The model under review builds one solid part; all positions refer to its coordinate system, in mm. Face numbers are marked on the shaded views. Give positions to 0.01 mm unless a question says otherwise; leave off trailing zeros. Order: outer loops, then holes, each group sorted by start corner. A loop starts at its lowest first (then second) coordinate and runs counter-clockwise, first axis right, second up. Notation, with made-up numbers: (-40, 72.25) - (14, 72.25) arc R23 cw to (14, 105.25) - close; hole circle Ø9 at (80, -26.75). An arc over 180 degrees is marked (long way). Answer as CSV lines item,"result". Start each with the question number.
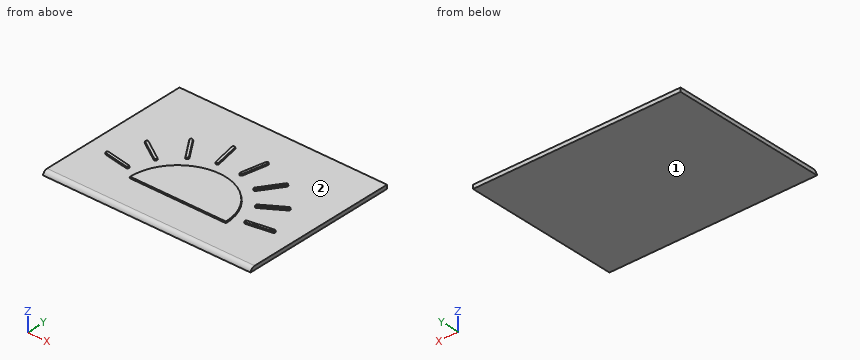
from build123d import *

# Parameters (mm, degrees)
SKETCH1_W                     = 129
SKETCH1_H                     = 97
BOSS_EXTRUDE1_DEPTH           = 2.4
FILLET1_R                     = 3
BOSS_EXTRUDE2_DEPTH           = 0.8
BOSS_EXTRUDE2_DRAFT           = 15
BOSS_EXTRUDE2_PROFILE_2_DEPTH = 0.8
BOSS_EXTRUDE2_PROFILE_2_DRAFT = 15
BOSS_EXTRUDE2_PROFILE_3_DEPTH = 0.8
BOSS_EXTRUDE2_PROFILE_3_DRAFT = 15
BOSS_EXTRUDE2_PROFILE_4_DEPTH = 0.8
BOSS_EXTRUDE2_PROFILE_4_DRAFT = 15
BOSS_EXTRUDE2_PROFILE_5_DEPTH = 0.8
BOSS_EXTRUDE2_PROFILE_5_DRAFT = 15
BOSS_EXTRUDE2_PROFILE_6_DEPTH = 0.8
BOSS_EXTRUDE2_PROFILE_6_DRAFT = 15
BOSS_EXTRUDE2_PROFILE_7_DEPTH = 0.8
BOSS_EXTRUDE2_PROFILE_7_DRAFT = 15
BOSS_EXTRUDE2_PROFILE_8_DEPTH = 0.8
BOSS_EXTRUDE2_PROFILE_8_DRAFT = 15
BOSS_EXTRUDE2_PROFILE_9_DEPTH = 0.8
BOSS_EXTRUDE2_PROFILE_9_DRAFT = 15


with BuildPart() as part:
    # Sketch1 → Boss-Extrude1 (new body)
    with BuildSketch(Plane.XY):
        with Locations((64.5, 48.5)):
            Rectangle(SKETCH1_W, SKETCH1_H)
    extrude(amount=BOSS_EXTRUDE1_DEPTH)

    # Fillet1
    # the kernel refuses this fillet: 3 mm, written as the material it takes off along each edge
    with BuildSketch(Plane(origin=(-7.348469228, 0, 2.4), x_dir=(0, 1.5674498735994488e-12, -1.0), z_dir=(1, 0, 0))) as fillet1_piece_1:
        with BuildLine():
            CenterArc((3, 2.939387691), FILLET1_R, 180, 78.463040967)
            Line((0, 2.939387691), (-0.06, 2.939387691))
            Line((-0.06, 2.939387691), (-0.06, 0))
            Line((-0.06, 0), (0, -0.06))
            ThreePointArc((0, -0.06), (1.2, -0.06), (2.388, -0.058787754))
            Line((2.388, -0.058787754), (2.4, 0))
        make_face()
    extrude(amount=143.696938457, mode=Mode.SUBTRACT)


with BuildPart() as boss_extrude2_tool:
    # Sketch2 → Boss-Extrude2 (with draft: the straight prism first)
    with BuildSketch(Plane.XY.offset(2.4)):
        with BuildLine():
            Line((34.5, 22), (94.5, 22))
            ThreePointArc((94.5, 22), (64.5, 52), (34.5, 22))
        make_face()
    extrude(amount=BOSS_EXTRUDE2_DEPTH)
    # Boss-Extrude2: the draft: its side faces are tilted about the plane it starts from
    boss_extrude2_sides = [boss_extrude2_tool.faces().sort_by_distance(p)[0] for p in [
        (64.5, 22, 2.8),
        (64.5, 52, 2.8),
    ]]
    draft(boss_extrude2_sides, Plane.XY.offset(2.4), BOSS_EXTRUDE2_DRAFT)


with BuildPart() as part_1:
    add(part.part)

    # Boss-Extrude2: add boss_extrude2_tool
    add(boss_extrude2_tool.part)


with BuildPart() as boss_extrude2_profile_2_tool:
    # Sketch2 → Boss-Extrude2 profile 2 (with draft: the straight prism first)
    with BuildSketch(Plane.XY.offset(2.4)):
        with BuildLine():
            ThreePointArc((12.971241145, 32.101337081), (11.812785214, 31.290177505), (12.623944789, 30.131721575))
            Line((12.623944789, 30.131721575), (27.396061084, 27.526998909))
            ThreePointArc((27.396061084, 27.526998909), (28.554517015, 28.338158485), (27.74335744, 29.496614416))
            Line((27.74335744, 29.496614416), (12.971241145, 32.101337081))
        make_face()
    extrude(amount=BOSS_EXTRUDE2_PROFILE_2_DEPTH)
    # Boss-Extrude2 profile 2: the draft: its side faces are tilted about the plane it starts from
    boss_extrude2_profile_2_sides = [boss_extrude2_profile_2_tool.faces().sort_by_distance(p)[0] for p in [
        (11.812785214, 31.290177505, 2.8),
        (20.010002937, 28.829360242, 2.8),
        (28.554517015, 28.338158485, 2.8),
        (20.357299292, 30.798975748, 2.8),
    ]]
    draft(boss_extrude2_profile_2_sides, Plane.XY.offset(2.4), BOSS_EXTRUDE2_PROFILE_2_DRAFT)


with BuildPart() as part_2:
    add(part_1.part)

    # Boss-Extrude2 profile 2: add boss_extrude2_profile_2_tool
    add(boss_extrude2_profile_2_tool.part)


with BuildPart() as boss_extrude2_profile_3_tool:
    # Sketch2 → Boss-Extrude2 profile 3 (with draft: the straight prism first)
    with BuildSketch(Plane.XY.offset(2.4)):
        with BuildLine():
            ThreePointArc((20.941185298, 51.323704776), (19.558613111, 51.026225117), (19.856092771, 49.64365293))
            Line((19.856092771, 49.64365293), (32.456481618, 41.505458972))
            ThreePointArc((32.456481618, 41.505458972), (33.839053805, 41.802938631), (33.541574146, 43.185510818))
            Line((33.541574146, 43.185510818), (20.941185298, 51.323704776))
        make_face()
    extrude(amount=BOSS_EXTRUDE2_PROFILE_3_DEPTH)
    # Boss-Extrude2 profile 3: the draft: its side faces are tilted about the plane it starts from
    boss_extrude2_profile_3_sides = [boss_extrude2_profile_3_tool.faces().sort_by_distance(p)[0] for p in [
        (33.839053805, 41.802938631, 2.8),
        (27.241379722, 47.254607797, 2.8),
        (19.558613111, 51.026225117, 2.8),
        (26.156287194, 45.574555951, 2.8),
    ]]
    draft(boss_extrude2_profile_3_sides, Plane.XY.offset(2.4), BOSS_EXTRUDE2_PROFILE_3_DRAFT)


with BuildPart() as part_3:
    add(part_2.part)

    # Boss-Extrude2 profile 3: add boss_extrude2_profile_3_tool
    add(boss_extrude2_profile_3_tool.part)


with BuildPart() as boss_extrude2_profile_4_tool:
    # Sketch2 → Boss-Extrude2 profile 4 (with draft: the straight prism first)
    with BuildSketch(Plane.XY.offset(2.4)):
        with BuildLine():
            ThreePointArc((35.751935726, 65.94085571), (34.362376894, 66.203774426), (34.099458177, 64.814215594))
            Line((34.099458177, 64.814215594), (42.549259048, 52.420633979))
            ThreePointArc((42.549259048, 52.420633979), (43.938817881, 52.157715263), (44.201736597, 53.547274095))
            Line((44.201736597, 53.547274095), (35.751935726, 65.94085571))
        make_face()
    extrude(amount=BOSS_EXTRUDE2_PROFILE_4_DEPTH)
    # Boss-Extrude2 profile 4: the draft: its side faces are tilted about the plane it starts from
    boss_extrude2_profile_4_sides = [boss_extrude2_profile_4_tool.faces().sort_by_distance(p)[0] for p in [
        (38.324358613, 58.617424786, 2.8),
        (43.938817881, 52.157715263, 2.8),
        (39.976836161, 59.744064902, 2.8),
        (34.362376894, 66.203774426, 2.8),
    ]]
    draft(boss_extrude2_profile_4_sides, Plane.XY.offset(2.4), BOSS_EXTRUDE2_PROFILE_4_DRAFT)


with BuildPart() as part_4:
    add(part_3.part)

    # Boss-Extrude2 profile 4: add boss_extrude2_profile_4_tool
    add(boss_extrude2_profile_4_tool.part)


with BuildPart() as boss_extrude2_profile_5_tool:
    # Sketch2 → Boss-Extrude2 profile 5 (with draft: the straight prism first)
    with BuildSketch(Plane.XY.offset(2.4)):
        with BuildLine():
            ThreePointArc((55.07749997, 73.657201755), (53.899181339, 74.4392281), (53.117154994, 73.260909469))
            Line((53.117154994, 73.260909469), (56.089347142, 58.558322151))
            ThreePointArc((56.089347142, 58.558322151), (57.267665773, 57.776295806), (58.049692118, 58.954614438))
            Line((58.049692118, 58.954614438), (55.07749997, 73.657201755))
        make_face()
    extrude(amount=BOSS_EXTRUDE2_PROFILE_5_DEPTH)
    # Boss-Extrude2 profile 5: the draft: its side faces are tilted about the plane it starts from
    boss_extrude2_profile_5_sides = [boss_extrude2_profile_5_tool.faces().sort_by_distance(p)[0] for p in [
        (53.899181339, 74.4392281, 2.8),
        (54.603251068, 65.90961581, 2.8),
        (57.267665773, 57.776295806, 2.8),
        (56.563596044, 66.305908096, 2.8),
    ]]
    draft(boss_extrude2_profile_5_sides, Plane.XY.offset(2.4), BOSS_EXTRUDE2_PROFILE_5_DRAFT)


with BuildPart() as part_5:
    add(part_4.part)

    # Boss-Extrude2 profile 5: add boss_extrude2_profile_5_tool
    add(boss_extrude2_profile_5_tool.part)


with BuildPart() as boss_extrude2_profile_6_tool:
    # Sketch2 → Boss-Extrude2 profile 6 (with draft: the straight prism first)
    with BuildSketch(Plane.XY.offset(2.4)):
        with BuildLine():
            ThreePointArc((75.882845006, 73.260909469), (75.100818661, 74.4392281), (73.92250003, 73.657201755))
            Line((73.92250003, 73.657201755), (70.950307882, 58.954614438))
            ThreePointArc((70.950307882, 58.954614438), (71.732334227, 57.776295806), (72.910652858, 58.558322151))
            Line((72.910652858, 58.558322151), (75.882845006, 73.260909469))
        make_face()
    extrude(amount=BOSS_EXTRUDE2_PROFILE_6_DEPTH)
    # Boss-Extrude2 profile 6: the draft: its side faces are tilted about the plane it starts from
    boss_extrude2_profile_6_sides = [boss_extrude2_profile_6_tool.faces().sort_by_distance(p)[0] for p in [
        (75.100818661, 74.4392281, 2.8),
        (72.436403956, 66.305908096, 2.8),
        (71.732334227, 57.776295806, 2.8),
        (74.396748932, 65.90961581, 2.8),
    ]]
    draft(boss_extrude2_profile_6_sides, Plane.XY.offset(2.4), BOSS_EXTRUDE2_PROFILE_6_DRAFT)


with BuildPart() as part_6:
    add(part_5.part)

    # Boss-Extrude2 profile 6: add boss_extrude2_profile_6_tool
    add(boss_extrude2_profile_6_tool.part)


with BuildPart() as boss_extrude2_profile_7_tool:
    # Sketch2 → Boss-Extrude2 profile 7 (with draft: the straight prism first)
    with BuildSketch(Plane.XY.offset(2.4)):
        with BuildLine():
            ThreePointArc((94.900541823, 64.814215594), (94.637623106, 66.203774426), (93.248064274, 65.94085571))
            Line((93.248064274, 65.94085571), (84.798263403, 53.547274095))
            ThreePointArc((84.798263403, 53.547274095), (85.061182119, 52.157715263), (86.450740952, 52.420633979))
            Line((86.450740952, 52.420633979), (94.900541823, 64.814215594))
        make_face()
    extrude(amount=BOSS_EXTRUDE2_PROFILE_7_DEPTH)
    # Boss-Extrude2 profile 7: the draft: its side faces are tilted about the plane it starts from
    boss_extrude2_profile_7_sides = [boss_extrude2_profile_7_tool.faces().sort_by_distance(p)[0] for p in [
        (94.637623106, 66.203774426, 2.8),
        (89.023163839, 59.744064902, 2.8),
        (85.061182119, 52.157715263, 2.8),
        (90.675641387, 58.617424786, 2.8),
    ]]
    draft(boss_extrude2_profile_7_sides, Plane.XY.offset(2.4), BOSS_EXTRUDE2_PROFILE_7_DRAFT)


with BuildPart() as part_7:
    add(part_6.part)

    # Boss-Extrude2 profile 7: add boss_extrude2_profile_7_tool
    add(boss_extrude2_profile_7_tool.part)


with BuildPart() as boss_extrude2_profile_8_tool:
    # Sketch2 → Boss-Extrude2 profile 8 (with draft: the straight prism first)
    with BuildSketch(Plane.XY.offset(2.4)):
        with BuildLine():
            ThreePointArc((109.143907229, 49.64365293), (109.441386889, 51.026225117), (108.058814702, 51.323704776))
            Line((108.058814702, 51.323704776), (95.458425854, 43.185510818))
            ThreePointArc((95.458425854, 43.185510818), (95.160946195, 41.802938631), (96.543518382, 41.505458972))
            Line((96.543518382, 41.505458972), (109.143907229, 49.64365293))
        make_face()
    extrude(amount=BOSS_EXTRUDE2_PROFILE_8_DEPTH)
    # Boss-Extrude2 profile 8: the draft: its side faces are tilted about the plane it starts from
    boss_extrude2_profile_8_sides = [boss_extrude2_profile_8_tool.faces().sort_by_distance(p)[0] for p in [
        (102.843712806, 45.574555951, 2.8),
        (109.441386889, 51.026225117, 2.8),
        (101.758620278, 47.254607797, 2.8),
        (95.160946195, 41.802938631, 2.8),
    ]]
    draft(boss_extrude2_profile_8_sides, Plane.XY.offset(2.4), BOSS_EXTRUDE2_PROFILE_8_DRAFT)


with BuildPart() as part_8:
    add(part_7.part)

    # Boss-Extrude2 profile 8: add boss_extrude2_profile_8_tool
    add(boss_extrude2_profile_8_tool.part)


with BuildPart() as boss_extrude2_profile_9_tool:
    # Sketch2 → Boss-Extrude2 profile 9 (with draft: the straight prism first)
    with BuildSketch(Plane.XY.offset(2.4)):
        with BuildLine():
            ThreePointArc((116.376055211, 30.131721575), (117.187214786, 31.290177505), (116.028758855, 32.101337081))
            Line((116.028758855, 32.101337081), (101.25664256, 29.496614416))
            ThreePointArc((101.25664256, 29.496614416), (100.445482985, 28.338158485), (101.603938916, 27.526998909))
            Line((101.603938916, 27.526998909), (116.376055211, 30.131721575))
        make_face()
    extrude(amount=BOSS_EXTRUDE2_PROFILE_9_DEPTH)
    # Boss-Extrude2 profile 9: the draft: its side faces are tilted about the plane it starts from
    boss_extrude2_profile_9_sides = [boss_extrude2_profile_9_tool.faces().sort_by_distance(p)[0] for p in [
        (108.642700708, 30.798975748, 2.8),
        (100.445482985, 28.338158485, 2.8),
        (108.989997063, 28.829360242, 2.8),
        (117.187214786, 31.290177505, 2.8),
    ]]
    draft(boss_extrude2_profile_9_sides, Plane.XY.offset(2.4), BOSS_EXTRUDE2_PROFILE_9_DRAFT)


with BuildPart() as part_9:
    add(part_8.part)

    # Boss-Extrude2 profile 9: add boss_extrude2_profile_9_tool
    add(boss_extrude2_profile_9_tool.part)


solid = part_9.part
Item 1: Clearance check with a flat-ended pin moving along its axis: pin 1 (2 mm diameter, centred on x = 32, y = 81, fed in from -Z). State where the tip first meets the part, or that it passes through.
Item 2: Take a section at B-B on y = 11. Write out the cut boundary in (x, z), and give its area (3 significant figures).
Item 3: Take a section at A-A on x = 64.5. Write out the cut boundary in (y, z).
Item 4: Mouldability with a two-part tool opening along X and no side actions: class the marked faces 1 and 2 as released by +X, released by -X, zero draft, split by the parting line, or undercut.
Item 5: Take a section at C-C on x = 103. Write out the cut boundary in (y, z), and give its area (3 significant figures).
Item 6: For line 1 along X through (y, z) = (46.5, 2.7); line 2 along Z through (x, y) = (116, 40); line 3 along X through (y, z) = (48.5, 2.6), list the stretches that pass through material, from the lowest coordinate up.
Data:
1,pin 1,"stops at z = 0"
2,outline,"(0, 0) - (129, 0) - (129, 2.4) - (0, 2.4) - close"
2,area,"310 mm^2"
3,outline,"(0, 0) - (97, 0) - (97, 2.4) - (52, 2.4) - (51.79, 3.2) - (22.21, 3.2) - (22, 2.4) - (2.94, 2.4) arc R3 ccw to start"
4,face 1,"zero draft"
4,face 2,"undercut"
5,outline,"(0, 0) - (97, 0) - (97, 2.4) - (48.06, 2.4) - (47.8, 3.2) - (45.93, 3.2) - (45.68, 2.4) - (29.8, 2.4) - (29.59, 3.2) - (27.99, 3.2) - (27.77, 2.4) - (2.94, 2.4) arc R3 ccw to start"
5,area,"234 mm^2"
6,line 1,"x = 24.87 to 28.26, 47.33 to 81.67, 100.74 to 104.13"
6,line 2,"z = 0 to 2.4"
6,line 3,"x = 21.73 to 25.21, 50.55 to 78.45, 103.79 to 107.27"
